from build123d import *

# Parameters (mm, degrees)
F0_R     = 12.5
F1_DEPTH = 7.25


with BuildPart() as f1:
    # F0 (on Top) → F1 (new body)
    with BuildSketch(Plane.XY):
        with BuildLine():
            ThreePointArc((0, 17.5), (5.125631, 5.125631), (17.5, 0))
            Line((17.5, 0), (101, 0))
            ThreePointArc((101, 0), (104.535534, 1.464466), (106, 5))
            Line((106, 5), (106, 30))
            ThreePointArc((106, 30), (104.535534, 33.535534), (101, 35))
            Line((101, 35), (17.5, 35))
            ThreePointArc((17.5, 35), (5.125631, 29.874369), (0, 17.5))
        make_face()
        with Locations((17.5, 17.5)):
            Circle(F0_R, mode=Mode.SUBTRACT)
    extrude(amount=F1_DEPTH)

    # F2 (on face) → F3 (revolve, cut)
    with BuildSketch(Plane.XY.offset(7.25)):
        with BuildLine():
            Line((42, 10.5), (42, 7.5))
            Line((42, 7.5), (43, 7.5))
            Line((43, 7.5), (45, 10.5))
            Line((45, 10.5), (45, 23.5))
            Line((45, 23.5), (48.25, 23.5))
            Line((48.25, 23.5), (48.25, 25))
            ThreePointArc((48.25, 25), (47.517767, 26.767767), (45.75, 27.5))
            Line((45.75, 27.5), (42, 27.5))
            Line((42, 27.5), (42, 23.5))
            Line((42, 23.5), (42, 10.5))
        make_face()
    revolve(axis=Axis((42, 15.5, 7.25), (0, 1, 0)), mode=Mode.SUBTRACT)

    # F2 (on face) → F4 (revolve, cut)
    with BuildSketch(Plane.XY.offset(7.25)):
        with BuildLine():
            Line((60, 10.5), (60, 7.5))
            Line((60, 7.5), (61, 7.5))
            Line((61, 7.5), (63, 10.5))
            Line((63, 10.5), (63, 23.5))
            Line((63, 23.5), (66.25, 23.5))
            Line((66.25, 23.5), (66.25, 25))
            ThreePointArc((66.25, 25), (65.517767, 26.767767), (63.75, 27.5))
            Line((63.75, 27.5), (60, 27.5))
            Line((60, 27.5), (60, 23.5))
            Line((60, 23.5), (60, 10.5))
        make_face()
    revolve(axis=Axis((60, 15.5, 7.25), (0, 1, 0)), mode=Mode.SUBTRACT)

    # F2 (on face) → F5 (revolve, cut)
    with BuildSketch(Plane.XY.offset(7.25)):
        with BuildLine():
            Line((78, 10.5), (78, 7.5))
            Line((78, 7.5), (79, 7.5))
            Line((79, 7.5), (81, 10.5))
            Line((81, 10.5), (81, 23.5))
            Line((81, 23.5), (84.25, 23.5))
            Line((84.25, 23.5), (84.25, 25))
            ThreePointArc((84.25, 25), (83.517767, 26.767767), (81.75, 27.5))
            Line((81.75, 27.5), (78, 27.5))
            Line((78, 27.5), (78, 23.5))
            Line((78, 23.5), (78, 10.5))
        make_face()
    revolve(axis=Axis((78, 17, 7.25), (0, -1, 0)), mode=Mode.SUBTRACT)

    # F2 (on face) → F6 (revolve, cut)
    with BuildSketch(Plane.XY.offset(7.25)):
        with BuildLine():
            Line((96, 10.5), (96, 7.5))
            Line((96, 7.5), (97, 7.5))
            Line((97, 7.5), (99, 10.5))
            Line((99, 10.5), (99, 23.5))
            Line((99, 23.5), (102.25, 23.5))
            Line((102.25, 23.5), (102.25, 25))
            ThreePointArc((102.25, 25), (101.517767, 26.767767), (99.75, 27.5))
            Line((99.75, 27.5), (96, 27.5))
            Line((96, 27.5), (96, 23.5))
            Line((96, 23.5), (96, 10.5))
        make_face()
    revolve(axis=Axis((96, 15.5, 7.25), (0, 1, 0)), mode=Mode.SUBTRACT)


solid = f1.part
Check sheet for the modelled part. Datum: model origin and axes. Units: mm. A direction names the side the tool comes from. Round coordinates to 2 decimals unless told otherwise and drop trailing zeros. Loops run counter-clockwise (first coordinate to the right, second up) from the corner with the lowest first, then second, coordinate; pieces in that order, holes last. Notation, with made-up numbers: (-5, 42.5) -> (54, 42.5) arc R4 cw to (54, 47.5) -> close; hole circle Ø3 at (-28.75, -2). An arc over 180 degrees is marked (long way). Put each result on its own line as item: value. Start each with the question number.
1. Access from +Z, -Z, +X, -X, +Y, -Y to the whole of each face (thin tool, end or side, straight path). Record for faces 1 (the face through (60.07, 17.09, 4.25)), 2 (the face through (60, 35, 4)).
2. Section check A-A (x = 11). Enter the section's corners in (y, z), plus the area to 3 significant figures.
3. Draft check along X on faces 3 (the face through (96, 23.5, 4)), 4 (the face through (64, 18, 0)), 5 (the face through (105, 33, 4)). Enter one of: +X half, -X half, draft (parallel to the pull), parting line (faces both ways), or undercut.
4. Section check C-C (x = 28). Enter the section's corners in (y, z).
5. Section check B-B (x = 96). Enter the section's corners in (y, z).
6. Scan lines: probe 1 along Y at (x, z) = (17.5, 4.25); probe 2 along Y at (x, z) = (77.5, 3.75); probe 3 along X at (y, z) = (14.5, 5.5). Record each from-to range of solid material in increasing order.
Findings:
1. face 1: +Z
1. face 2: +Z, -Z, +X, -X, +Y
2. outline: (1.25, 0) -> (6.82, 0) -> (6.82, 7.25) -> (1.25, 7.25) -> close; (28.18, 0) -> (33.75, 0) -> (33.75, 7.25) -> (28.18, 7.25) -> close
2. area: 80.8 mm^2
3. face 3: undercut
3. face 4: draft
3. face 5: +X half
4. outline: (0, 0) -> (10.72, 0) -> (10.72, 7.25) -> (0, 7.25) -> close; (24.28, 0) -> (35, 0) -> (35, 7.25) -> (24.28, 7.25) -> close
5. outline: (0, 0) -> (35, 0) -> (35, 7.25) -> (27.5, 7.25) -> (27.5, 3.5) arc R2.5 cw to (25, 1) -> (23.5, 1) -> (23.5, 4.25) -> (10.5, 4.25) -> (7.5, 6.25) -> (7.5, 7.25) -> (0, 7.25) -> close
6. probe 1: y = 0 to 5, 30 to 35
6. probe 2: y = 0 to 23.5, 27.5 to 35
6. probe 3: x = 0.26 to 5.37, 29.63 to 39.56, 44.44 to 57.56, 62.44 to 75.56, 80.44 to 93.56, 98.44 to 106
